Here's how the part is built. I have some questions about the finished solid (model axes, mm). A direction names the side the tool comes from. Round coordinates to 2 decimals unless told otherwise and drop trailing zeros. Loops run counter-clockwise (first coordinate to the right, second up) from the corner with the lowest first, then second, coordinate; pieces in that order, holes last. Notation, with made-up numbers: M 53,-4.5 L 112,-4.5 A35 ccw 112,29.5 Z; hole C -35.75,68.5 d5. An arc over 180 degrees is marked long. Use a Markdown table: item, result.
Autodesk Inventor part; units mm, degrees
ref_plane "Arbeitsebene1" through (0, 0, 0) normal (1, 0, 0) x (0, 0, -1)
ref_plane "YZ Plane" through (0, 0, 0) normal (1, 0, 0) x (0, 1, 0)
ref_plane "XZ Plane" through (0, 0, 0) normal (0, 1, 0) x (-1, 0, 0)
ref_plane "Arbeitsebene1" through (0, 0, 0) normal (1, 0, 0) x (0, 0, -1)
sketch "Skizze1" plane through (0, 0, 0) normal (1, 0, 0) x (0, 0, -1)
  circle A0 centre (0, 0) radius 5.5
  line L0 (-24.52, 0) -> (24.52, 0) construction
  line L1 (0, -23.5528) -> (0, 22.3555) construction
  line L2 (8.89, -5.5) -> (-8.89, -5.5) construction
  line L3 (-8.89, -5.5) -> (-8.89, 5.5) construction
  line L4 (-8.89, 5.5) -> (8.89, 5.5) construction
  line L5 (8.89, 5.5) -> (8.89, -5.5) construction
  circle A1 centre (8.89, 5.5) radius 1.2
  circle A2 centre (-8.89, 5.5) radius 1.2
  arc A3 (-15.3, 0) -> (14.8761, 3.5767) centre (0, 0) ccw
  arc A4 (4.4, 3.3) -> (-4.4, 3.3) centre (0, 0) ccw
  circle A5 centre (8.89, -5.5) radius 1.2
  circle A6 centre (-8.89, -5.5) radius 1.2
  line L6 (-5.89, -5.5) -> (-5.89, 5.5)
  arc A7 (-5.89, 5.5) -> (-11.89, 5.5) centre (-8.89, 5.5) ccw
  arc A8 (11.89, 5.5) -> (5.89, 5.5) centre (8.89, 5.5) ccw
  line L7 (5.89, -5.5) -> (5.89, 5.5)
  circle A9 centre (8.89, -5.5) radius 2.15
  circle A10 centre (8.89, 5.5) radius 2.15
  circle A11 centre (-8.89, 5.5) radius 2.15
  circle A12 centre (0, 0) radius 11 construction
  circle A13 centre (-11, 0) radius 1.6
  circle A14 centre (11, 0) radius 1.6
  arc A15 (-11.89, -5.5) -> (-5.89, -5.5) centre (-8.89, -5.5) ccw
  arc A16 (5.89, -5.5) -> (11.89, -5.5) centre (8.89, -5.5) ccw
  line L8 (5.5, 0) -> (5.5, 14.2773)
  line L9 (-5.5, 0) -> (-5.5, 14.2773)
  arc A17 (15.3, 0) -> (5.5, 14.2773) centre (0, 0) ccw
  arc A18 (-5.5, 14.2773) -> (-15.3, 0) centre (0, 0) ccw
  line L10 (11.89, -5.5) -> (11.89, -3.1258)
  line L11 (11.89, 3.1258) -> (11.89, 5.5)
  line L12 (-11.89, -5.5) -> (-11.89, -3.1258)
  line L13 (-11.89, 3.1258) -> (-11.89, 5.5)
  circle A19 centre (11, 0) radius 3.25
  circle A20 centre (-11, 0) radius 3.25
  circle A21 centre (-8.89, -5.5) radius 2.15
  dimension "d2" = 11
  dimension "d19" = 11
  dimension "d20" = 17.78
  dimension "d22" = 2.4
  dimension "d29" = 15.3
  dimension "d30" = 5.5
  dimension "d38" = 3
  dimension "d52" = 22
  dimension "d53" = 3.2
  dimension "d55" = 6.5
  dimension "d60" = 4.3
extrude "Extrusion7" add sketch "Skizze1" along normal blind 3.2 contours L8 A17 A3 A18 L9 A0 | A6 | A15 L12 A20 L13 A7 L6 | A20 | L11 A19 L10 A16 L7 A8 | A19 | A21
extrude "Extrusion3" add sketch "Skizze1" against normal blind 5 from surface at 0 contours A6 | A15 L12 A20 L13 A7 L6 | L11 A19 L10 A16 L7 A8 | A21
extrude "Extrusion4" add sketch "Skizze1" against normal blind 3 from surface at -5 contours A15 L12 A20 L13 A7 L6 | L11 A19 L10 A16 L7 A8 | A9 | A10 | A11 | A21
sketch "Skizze2" plane through (3.2, 0, 0) normal (1, 0, 0) x (0, 0, -1)
  circle A0 centre (0, 0) radius 8.25
  dimension "d57" = 16.5
extrude "Extrusion9" cut sketch "Skizze2" against normal blind 1.2
properties part number "AS5047DEnclosureV2"
1. Imagine slicing it at D-D, the plane z = 2. Write out the boundary of the cut face in (x, y), then the cut area to 3 significant figures.
Answer sheet:
| item | result |
|---|---|
| outline | M 0,-15.17 L 3.2,-15.17 L 3.2,-8 L 2,-8 L 2,-5.12 L 0,-5.12 Z |
| area | 28.7 mm2 |
2. We'd pull the mould along Z, two halves only. Please class faces 1 (the face through (-0.96, -7.31, -10.05)), 2 (the face through (-4, 4, 11.89)), 3 (the face through (-8, 0.1, 7.6)), 4 (the face through (-4, -4, -11.89)): +Z half, -Z half, draft (parallel to the pull), parting line (faces both ways), or undercut.
Answer sheet:
| item | result |
|---|---|
| face 1 | undercut |
| face 2 | +Z half |
| face 3 | draft |
| face 4 | -Z half |
3. Which directions (+Z, -Z, +X, -X, +Y, -Y) give clear straight access to the entire face, cutting with the end or side of a thin tool? Please do faces 5 (the face through (-5, -5, 9)), 6 (the face through (2, -6, 0)), 7 (the face through (-3.94, -8.5, 8.96)).
Answer sheet:
| item | result |
|---|---|
| face 5 | -X |
| face 6 | +X |
| face 7 | -X, -Y |
4. Imagine slicing it at C-C, the plane x = -6.75. Write out the boundary of the cut face in (y, z).
Answer sheet:
| item | result |
|---|---|
| outline | M -5.5,-11.89 L -3.13,-11.89 A3.25 cw long 3.13,-11.89 L 5.5,-11.89 A3 ccw 5.5,-5.89 L -5.5,-5.89 A3 ccw Z; M -5.5,5.89 L 5.5,5.89 A3 ccw 5.5,11.89 L 3.13,11.89 A3.25 cw long -3.13,11.89 L -5.5,11.89 A3 ccw Z; hole C -5.5,-8.89 d2.4; hole C -5.5,8.89 d2.4; hole C 5.5,-8.89 d2.4; hole C 5.5,8.89 d2.4 |
5. I need wall thicknesses on probe 1 along Z at (x, y) = (-1.5, 0); probe 2 along Z at (x, y) = (-1.5, 7.25); probe 3 along Y at (x, z) = (-6, 8.89). Which ranges of each line are inside material? Lowest first, please. Write a range as from..to.
Answer sheet:
| item | result |
|---|---|
| probe 1 | -7.75..-5.89, 5.89..7.75 |
| probe 2 | -11.33..-10.14, -7.64..-6.45, 6.45..7.64, 10.14..11.33 |
| probe 3 | -8.5..-6.7, -4.3..-2.47, 2.47..4.3, 6.7..8.5 |
6. Imagine slicing it at B-B, the plane x = -1.25. Write out the boundary of the cut face in (y, z), then the cut area to 3 significant figures.
Answer sheet:
| item | result |
|---|---|
| outline | M -5.5,-11.89 L -3.13,-11.89 A3.25 cw long 3.13,-11.89 L 5.5,-11.89 A3 ccw 5.5,-5.89 L -5.5,-5.89 A3 ccw Z; M -5.5,5.89 L 5.5,5.89 A3 ccw 5.5,11.89 L 3.13,11.89 A3.25 cw long -3.13,11.89 L -5.5,11.89 A3 ccw Z; hole C -5.5,-8.89 d4.3; hole C 5.5,-8.89 d4.3; hole C 5.5,8.89 d4.3 |
| area | 100 mm2 |
7. For pin 1 Ø4 at (x, z) = (-6, 7) entering from +Y; pin 2 Ø1.6 at (x, y) = (1.5, 7.5) entering from -Z (3 decimals); pin 3 Ø1 at (x, z) = (-4, 5) entering from +Y; pin 4 Ø2.5 at (x, y) = (-2.5, 1) entering from -Z, each with a flat end and sliding along its axis, tell me the tip position at first contact or that it passes through.
Answer sheet:
| item | result |
|---|---|
| pin 1 | y = 8.5 |
| pin 2 | z = -13.755 |
| pin 3 | through |
| pin 4 | z = -8.65 |
8. Imagine slicing it at A-A, the plane z = 8.89. Write out the boundary of the cut face in (x, y).
Answer sheet:
| item | result |
|---|---|
| outline | M -8,-8.5 L 0,-8.5 L 0,-12.45 L 3.2,-12.45 L 3.2,3.35 L -5,3.35 L -5,4.3 L -8,4.3 L -8,2.47 L 0,2.47 L 0,-2.47 L -8,-2.47 L -8,-4.3 L -5,-4.3 L -5,-6.7 L -8,-6.7 Z; M -8,6.7 L -5,6.7 L -5,7.65 L 3.2,7.65 L 3.2,12.45 L 0,12.45 L 0,8.5 L -8,8.5 Z |
